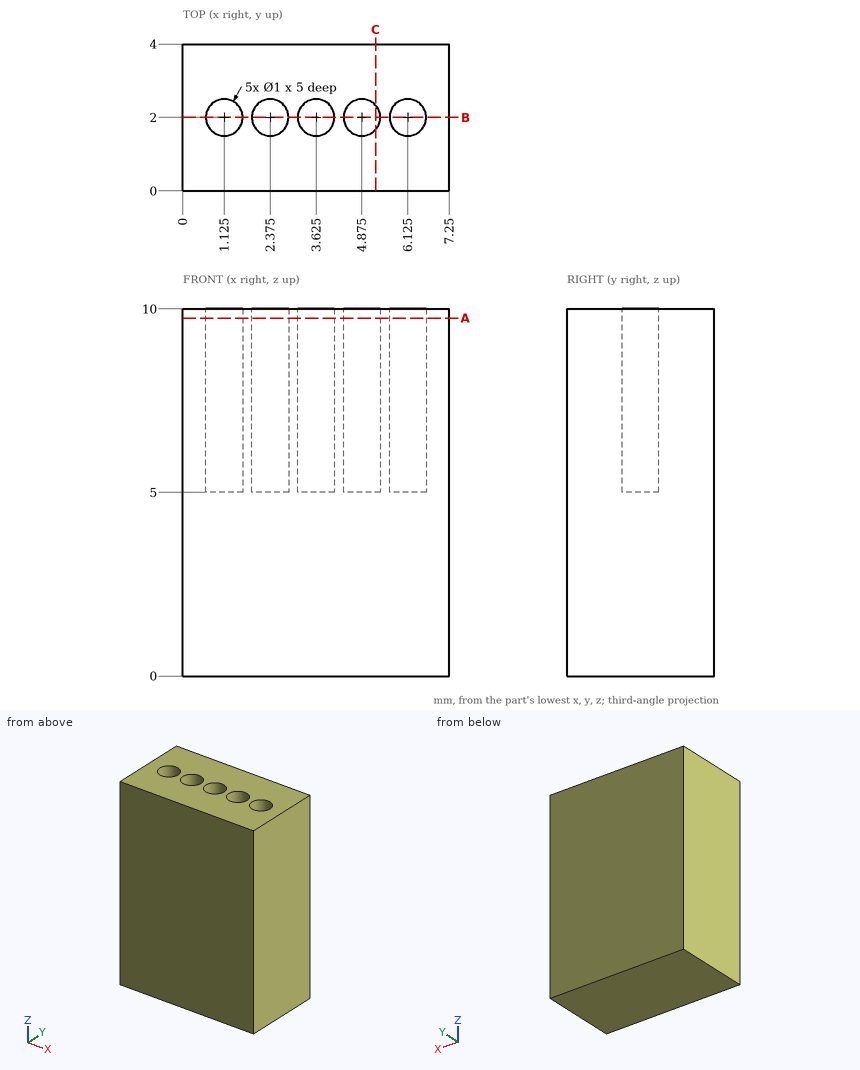
Drawing for the job (mm, zero at the part's lowest x, y, z). Give positions to 0.01 mm unless a question says otherwise; leave off trailing zeros. Order: outer loops, then holes, each group sorted by start corner. A loop starts at its lowest first (then second) coordinate and runs counter-clockwise, first axis right, second up. Notation, with made-up numbers: M 87.25,-28 L 93.25,-28 A32 cw 93.25,3 Z; hole C -16.75,-39.75 d6. An arc over 180 degrees is marked long. Put each result on its own line as item: value.
Item 1: Probe line 1 (X direction, y = 1.6, z = 8.5) (3 decimals); line 2 (Y direction, x = 1, z = 5.5); line 3 (Y direction, x = 0.75, z = 8.5). List the from-to ranges inside material, lowest first. Write a range as [from, to].
From the geometry:
line 1: x = [0, 0.825], [1.425, 2.075], [2.675, 3.325], [3.925, 4.575], [5.175, 5.825], [6.425, 7.25]
line 2: y = [0, 1.52], [2.48, 4]
line 3: y = [0, 1.67], [2.33, 4]
Item 2: Slice it at B-B, the plane y = 2. Write the cut outline in (x, z) (3 decimals).
From the geometry:
outline: M 0,0 L 7.25,0 L 7.25,10 L 6.625,10 L 6.625,5 L 5.625,5 L 5.625,10 L 5.375,10 L 5.375,5 L 4.375,5 L 4.375,10 L 4.125,10 L 4.125,5 L 3.125,5 L 3.125,10 L 2.875,10 L 2.875,5 L 1.875,5 L 1.875,10 L 1.625,10 L 1.625,5 L 0.625,5 L 0.625,10 L 0,10 Z
Item 3: Flat gauge pins, fed straight in: pin 1 Ø0.5 at (x, y) = (6, 2) entering from +Z; pin 2 Ø0.5 at (x, y) = (1.5, 2) entering from +Z. Where does each tip first touch, or does it go through?
From the geometry:
pin 1: stops at z = 5
pin 2: stops at z = 10
Item 4: Slice it at A-A, the plane z = 9.75. Write the cut outline in (x, y) (3 decimals), plus the area to 3 significant figures.
From the geometry:
outline: M 0,0 L 7.25,0 L 7.25,4 L 0,4 Z; hole C 1.125,2 d1; hole C 2.375,2 d1; hole C 3.625,2 d1; hole C 4.875,2 d1; hole C 6.125,2 d1
area: 25.1 mm2
Item 5: Slice it at C-C, the plane x = 5.25. Write the cut outline in (y, z), plus the area to 3 significant figures.
From the geometry:
outline: M 0,0 L 4,0 L 4,10 L 2.33,10 L 2.33,5 L 1.67,5 L 1.67,10 L 0,10 Z
area: 36.7 mm2
